Read the model definition and answer for the solid it produces. Units are mm, in the model's axes. Round coordinates to 2 decimals unless told otherwise and drop trailing zeros. Order: outer loops, then holes, each group sorted by start corner. A loop starts at its lowest first (then second) coordinate and runs counter-clockwise, first axis right, second up. Notation, with made-up numbers: (-34.5, -16) -> (21.5, -16) arc R20 ccw to (21.5, -3) -> close; hole circle Ø2 at (88.25, 40). An arc over 180 degrees is marked (long way). Answer as a JSON object with one key per item and string values. Group by question number.
Item 1: Section A-A, the plane y = -68 is taken. Write down the section's boundary in (x, z), plus the area to 3 significant figures.
Item 2: Consider probe 1 along X at (y, z) = (-63, 0.5); probe 2 along X at (y, z) = (-61, 0.3); probe 3 along Y at (x, z) = (32, 0.2). Determine where each line is inside the solid, lowest interval first. Write a range as from..to.
Item 3: Section B-B, the plane z = 0.4 is taken. Write down the section's boundary in (x, y).
Autodesk Inventor part; units mm, degrees
ref_plane "YZ Plane" through (0, 0, 0) normal (1, 0, 0) x (0, 1, 0)
ref_plane "XZ Plane" through (0, 0, 0) normal (0, 1, 0) x (-1, 0, 0)
ref_plane "XY Plane" through (0, 0, 0) normal (0, 0, 1) x (1, 0, 0)
ref_plane "Work Plane1" through (0, 0, 0) normal (0, 0, 1) x (1, 0, 0)
sketch "Sketch1" plane through (0, 0, 0) normal (0, 0, 1) x (1, 0, 0)
  line L0 (84.5, 12.4325) -> (84.5, -11.5675)
  line L1 (84.5, -11.5675) -> (72.5, -11.5675)
  line L2 (72.5, -11.5675) -> (72.5, 4.5875)
  circle A0 centre (69.5, 4.5875) radius 3
  line L3 (72.5, 4.5875) -> (72.5, 12.4325)
  line L4 (72.5, 12.4325) -> (84.5, 12.4325)
  arc A1 (105.5, 4.2836) -> (105.5, 4.8914) centre (108.4846, 4.5875) ccw
  line L5 (105.5, 4.2836) -> (105.5, -11.5675)
  line L6 (105.5, -11.5675) -> (93.5, -11.5675)
  line L7 (93.5, -11.5675) -> (93.5, 12.4325)
  line L8 (93.5, 12.4325) -> (105.5, 12.4325)
  line L9 (105.5, 12.4325) -> (105.5, 4.8914)
  circle A2 centre (108.4462, 27.5) radius 3
  circle A3 centre (69.5, 27.5) radius 3
  circle A4 centre (89, 0.9661) radius 3
  circle A5 centre (89, 29.5) radius 3
  arc A6 (175, 0) -> (178, -3) centre (175, -3) ccw
  line L10 (175, 0) -> (115.0397, 0)
  line L11 (65.5, 33.8) -> (65.5, 0)
  line L12 (65.5, 0) -> (65.1397, 0)
  arc A7 (0, -3) -> (3, 0) centre (3, -3) ccw
  line L13 (0, -3) -> (0, -25.75)
  arc A8 (3, -28.75) -> (0, -25.75) centre (3, -25.75) ccw
  line L14 (3, -28.75) -> (62.9603, -28.75)
  arc A9 (178, -25.75) -> (175, -28.75) centre (175, -25.75) ccw
  line L15 (178, -25.75) -> (178, -3)
  circle A10 centre (3, -25.75) radius 2.3
  circle A11 centre (3, -3) radius 2.3
  circle A12 centre (3, -74.8889) radius 2.3
  line L16 (0, 0) -> (6, 0)
  line L17 (0, -77.8889) -> (0, 0)
  line L18 (0, -77.8889) -> (6, -77.8889)
  line L19 (6, -71.8889) -> (6, -77.8889)
  line L20 (6, -71.8889) -> (1.6, -71.8889)
  line L21 (1.6, -71.8889) -> (1.6, -56.7889)
  line L22 (1.6, -56.7889) -> (3, -56.7889)
  line L23 (3, -28.75) -> (3, -56.7889)
  line L24 (3, -28.75) -> (6, -28.75)
  line L25 (6, -28.75) -> (6, -22.75)
  line L26 (6, -22.75) -> (3, -22.75)
  line L27 (3, -6) -> (3, -22.75)
  line L28 (3, -6) -> (6, -6)
  line L29 (6, -6) -> (6, 0)
  circle A13 centre (175, -3) radius 2.3
  circle A14 centre (175, -25.75) radius 2.3
  line L30 (175, -28.75) -> (175, -71.8889)
  line L31 (175, -6) -> (175, -22.75)
  line L32 (175, -71.8889) -> (172, -71.8889)
  line L33 (172, -71.8889) -> (172, -77.8889)
  line L34 (178, -77.8889) -> (172, -77.8889)
  line L35 (178, -77.8889) -> (178, 0)
  line L36 (178, 0) -> (172, 0)
  line L37 (172, 0) -> (172, -6)
  line L38 (172, -6) -> (175, -6)
  line L39 (175, -22.75) -> (172, -22.75)
  line L40 (172, -22.75) -> (172, -28.75)
  line L41 (172, -28.75) -> (175, -28.75)
  circle A15 centre (175, -74.8889) radius 2.3
  line L42 (156.2, -70.4889) -> (156.2, -59.9889)
  line L43 (166.7, -59.9889) -> (156.2, -59.9889)
  line L44 (166.7, -59.9889) -> (166.7, -70.4889)
  line L45 (156.2, -70.4889) -> (166.7, -70.4889)
  line L46 (149, -59.8889) -> (149, -70.8889)
  line L47 (149, -70.8889) -> (136.35, -70.8889)
  line L48 (136.35, -70.8889) -> (136.35, -59.8889)
  line L49 (136.35, -59.8889) -> (149, -59.8889)
  line L50 (135, -53.8889) -> (135, -71.8889)
  line L51 (135, -71.8889) -> (175, -71.8889)
  line L52 (175, -71.8889) -> (175, -53.8889)
  line L53 (175, -53.8889) -> (135, -53.8889)
  circle A16 centre (137.85, -56.7389) radius 1.5
  circle A17 centre (172.15, -56.7389) radius 1.5
  line L54 (31.25, -62.8889) -> (31.25, -73.8889)
  line L55 (31.25, -73.8889) -> (57.25, -73.8889)
  line L56 (57.25, -73.8889) -> (57.25, -62.8889)
  line L57 (57.25, -62.8889) -> (31.25, -62.8889)
  line L58 (3, -56.7889) -> (23.3, -56.7889)
  line L59 (23.3, -56.7889) -> (23.3, -59.8889)
  line L60 (23.3, -59.8889) -> (23.3, -65.1889)
  line L61 (3, -71.8889) -> (23.3, -71.8889)
  line L62 (23.3, -61.8889) -> (23.3, -74.8889)
  line L63 (30.25, -61.8889) -> (30.25, -74.8889)
  line L64 (30.25, -74.8889) -> (58.25, -74.8889)
  line L65 (58.25, -74.8889) -> (58.25, -61.8889)
  line L66 (58.25, -61.8889) -> (30.25, -61.8889)
  line L67 (150, -58.8889) -> (150, -71.8889)
  line L68 (150, -71.8889) -> (135.35, -71.8889)
  line L69 (135.35, -71.8889) -> (135.35, -58.8889)
  line L70 (135.35, -58.8889) -> (150, -58.8889)
  line L71 (155.2, -58.9889) -> (155.2, -71.4889)
  line L72 (155.2, -71.4889) -> (167.7, -71.4889)
  line L73 (167.7, -71.4889) -> (167.7, -58.9889)
  line L74 (167.7, -58.9889) -> (155.2, -58.9889)
  line L75 (0, -28.75) -> (178, -28.75)
  line L76 (178, -28.75) -> (178, -77.8889)
  line L77 (178, -77.8889) -> (0, -77.8889)
  line L78 (0, -77.8889) -> (0, -28.75)
  line L79 (131.125, -21.1625) -> (131.125, -7.525)
  arc A18 (134.125, -4.525) -> (131.125, -7.525) centre (134.125, -7.525) ccw
  line L80 (134.125, -4.525) -> (155.95, -4.525)
  arc A19 (158.95, -7.525) -> (155.95, -4.525) centre (155.95, -7.525) ccw
  line L81 (158.95, -7.525) -> (158.95, -21.1625)
  arc A20 (155.95, -24.1625) -> (158.95, -21.1625) centre (155.95, -21.1625) ccw
  line L82 (155.95, -24.1625) -> (134.125, -24.1625)
  arc A21 (131.125, -21.1625) -> (134.125, -24.1625) centre (134.125, -21.1625) ccw
  line L83 (46.875, -7.5875) -> (46.875, -21.225)
  arc A22 (43.875, -24.225) -> (46.875, -21.225) centre (43.875, -21.225) ccw
  line L84 (43.875, -24.225) -> (22.05, -24.225)
  arc A23 (19.05, -21.225) -> (22.05, -24.225) centre (22.05, -21.225) ccw
  line L85 (19.05, -21.225) -> (19.05, -7.5875)
  arc A24 (22.05, -4.5875) -> (19.05, -7.5875) centre (22.05, -7.5875) ccw
  line L86 (22.05, -4.5875) -> (43.875, -4.5875)
  arc A25 (46.875, -7.5875) -> (43.875, -4.5875) centre (43.875, -7.5875) ccw
  line L87 (112.5, 0) -> (112.5, 33.8)
  line L88 (112.5, 33.8) -> (65.5, 33.8)
  arc A26 (115.0397, -28.75) -> (112.8603, -28.75) centre (113.95, -26.5) ccw
  line L89 (115.0397, -28.75) -> (175, -28.75)
  arc A27 (112.8603, 0) -> (115.0397, 0) centre (113.95, -2.25) ccw
  line L90 (112.8603, 0) -> (112.5, 0)
  arc A28 (62.9603, 0) -> (65.1397, 0) centre (64.05, -2.25) ccw
  line L91 (62.9603, 0) -> (3, 0)
  arc A29 (65.1397, -28.75) -> (62.9603, -28.75) centre (64.05, -26.5) ccw
  line L92 (65.1397, -28.75) -> (112.8603, -28.75)
  point P0 (168.4, -53.8889)
  point P1 (135.35, -71.8889)
  point P2 (6, -25.75)
  point P3 (3, -28.75)
  dimension "d0" = 1
  dimension "d1" = 1
  dimension "d2" = 1
extrude "Extrusion1" add sketch "Sketch1" along normal blind 0.6 contours L35 L34 L33 L32 L30 L75 | L30 L53 L50 L51 L33 L77 L19 L61 L62 L60 L59 L58 L23 L14 L75 L41 | L30 L32 L51 L67 L70 L69 L50 L53 | L18 L17 L75 L23 L22 L21 L20 L19 | L20 L21 L22 L58 L59 L60 L62 L61 | A12 | A15 | A16 | A17
sketch "Sketch2" plane through (0, 0, 0.6) normal (0, 0, 1) x (1, 0, 0)
  circle A0 centre (3, -25.75) radius 2.3
  circle A1 centre (3, -3) radius 2.3
  circle A2 centre (3, -74.8889) radius 2.3
  line L0 (0, 0) -> (6, 0)
  line L1 (0, -77.8889) -> (0, 0)
  line L2 (0, -77.8889) -> (6, -77.8889)
  line L3 (6, -71.8889) -> (6, -77.8889)
  line L4 (6, -71.8889) -> (1.6, -71.8889)
  line L5 (1.6, -71.8889) -> (1.6, -56.7889)
  line L6 (1.6, -56.7889) -> (3, -56.7889)
  line L7 (3, -28.75) -> (3, -56.7889)
  line L8 (3, -28.75) -> (6, -28.75)
  line L9 (6, -28.75) -> (6, -22.75)
  line L10 (6, -22.75) -> (3, -22.75)
  line L11 (3, -6) -> (3, -22.75)
  line L12 (3, -6) -> (6, -6)
  line L13 (6, -6) -> (6, 0)
  circle A3 centre (175, -3) radius 2.3
  circle A4 centre (175, -25.75) radius 2.3
  line L14 (175, -28.75) -> (175, -71.8889)
  line L15 (175, -6) -> (175, -22.75)
  line L16 (175, -71.8889) -> (172, -71.8889)
  line L17 (172, -71.8889) -> (172, -77.8889)
  line L18 (178, -77.8889) -> (172, -77.8889)
  line L19 (178, -77.8889) -> (178, 0)
  line L20 (178, 0) -> (172, 0)
  line L21 (172, 0) -> (172, -6)
  line L22 (172, -6) -> (175, -6)
  line L23 (175, -22.75) -> (172, -22.75)
  line L24 (172, -22.75) -> (172, -28.75)
  line L25 (172, -28.75) -> (175, -28.75)
  circle A5 centre (175, -74.8889) radius 2.3
hole "Hole1" at (3, -74.8889, 0.6) at (175, -74.8889, 0.6) direction (0, 0, -1) diameter 3.6 end through all countersink diameter 6 countersink angle 90
properties part number "ceil_front" material "ABS Plastic"
Values found:
{
 "1": {"outline": "(0, 0) -> (30.25, 0) -> (30.25, 0.6) -> (0, 0.6) -> close; (58.25, 0) -> (135.35, 0) -> (135.35, 0.6) -> (58.25, 0.6) -> close; (150, 0) -> (155.2, 0) -> (155.2, 0.6) -> (150, 0.6) -> close; (167.7, 0) -> (178, 0) -> (178, 0.6) -> (167.7, 0.6) -> close", "area": "73.7 mm2"},
 "2": {"probe 1": "0..30.25, 58.25..135.35, 150..155.2, 167.7..178", "probe 2": "0..135.35, 150..155.2, 167.7..178", "probe 3": "-77.89..-74.89, -61.89..-28.75"},
 "3": {"outline": "(0, -77.89) -> (178, -77.89) -> (178, -28.75) -> (0, -28.75) -> close; hole circle Ø5.6 at (3, -74.89); hole (30.25, -74.89) -> (58.25, -74.89) -> (58.25, -61.89) -> (30.25, -61.89) -> close; hole (135.35, -71.89) -> (150, -71.89) -> (150, -58.89) -> (135.35, -58.89) -> close; hole (155.2, -71.49) -> (167.7, -71.49) -> (167.7, -58.99) -> (155.2, -58.99) -> close; hole circle Ø5.6 at (175, -74.89)"}
}
